```python
from build123d import *

# Parameters (mm, degrees)
ESTRUSIONE_ESTRUSIONE1_DEPTH = 5
SCHIZZO2_R                   = 2
TAGLIO_ESTRUSIONE1_DEPTH     = 5
SCHIZZO4_R                   = 4.75
TAGLIO_ESTRUSIONE2_DEPTH     = 10


with BuildPart() as part:
    # Schizzo1 → Estrusione-Estrusione1 (new body)
    with BuildSketch(Plane.XY):
        with BuildLine():
            Line((0, 145), (0, 120))
            ThreePointArc((0, 120), (-20.689655172, 118.2029533), (-40.759639069, 112.865636147))
            Line((-40.759639069, 112.865636147), (-49.251230542, 136.379310345))
            ThreePointArc((-49.251230542, 136.379310345), (-25, 142.828568571), (0, 145))
        make_face()
    extrude(amount=ESTRUSIONE_ESTRUSIONE1_DEPTH)

    # Schizzo2 → Taglio-Estrusione1 (cut)
    with BuildSketch(Plane.XY.offset(5)):
        with Locations((-38.032134419, 134.73513555)):
            Circle(SCHIZZO2_R)
        with Locations((-9.993620414, 139.642857143)):
            Circle(SCHIZZO2_R)
    extrude(amount=-TAGLIO_ESTRUSIONE1_DEPTH, mode=Mode.SUBTRACT)

    # Raccordo1
    # an asymmetric fillet: 20, 15 mm, written as the material it takes off along each edge
    with BuildSketch(Plane(origin=(-40.759639069, 112.865636147, -44.567563269), x_dir=(-0.3396636589081028, 0.9405469678953624, 0), z_dir=(0, 0, 1))) as raccordo1_piece_1:
        with BuildLine():
            Bezier((13.510299228, 0), (1.338953576, 0), (-1.324178464, -17.777777778), weights=[1, 0.757676761, 1])
            ThreePointArc((-1.324178464, -17.777777778), (-0.331502507, -8.913512654), (0, 0))
            Line((0, 0), (13.510299228, 0))
        make_face()
    extrude(amount=94.135126538, mode=Mode.SUBTRACT)

    # Raccordo2
    # an asymmetric fillet: 20, 15 mm, written as the material it takes off along each edge
    with BuildSketch(Plane(origin=(0, 120, -44.567563269), x_dir=(-0.9972374791061684, -0.07427927211527091, 0), z_dir=(0, 0, 1))) as raccordo2_piece_1:
        with BuildLine():
            Bezier((17.827025308, 0), (-0.099456497, -1.335254689), (-1.003535193, -13.472976744), weights=[1, 0.757676761, 1])
            Line((-1.003535193, -13.472976744), (0, 0))
            ThreePointArc((0, 0), (8.913512654, -0.331502507), (17.827025308, 0))
        make_face()
    extrude(amount=94.135126538, mode=Mode.SUBTRACT)

    # Schizzo4 → Taglio-Estrusione2 (cut)
    with BuildSketch(Plane.XY.offset(5)):
        with Locations((-22.24137931, 127.068174798)):
            Circle(SCHIZZO4_R)
    extrude(amount=-TAGLIO_ESTRUSIONE2_DEPTH, mode=Mode.SUBTRACT)


solid = part.part
```
Source: CAD feature listing. Evaluate the final solid. Frame: model axes, mm. Round coordinates to 2 decimals unless told otherwise and drop trailing zeros. Loops run counter-clockwise (first coordinate to the right, second up) from the corner with the lowest first, then second, coordinate; pieces in that order, holes last.
1. Mould query, pull axis Y, two halves, no side actions, for faces 1 (the cylindrical face through (-9.07, 137.87, 2.54)), 2 (the cylindrical face through (-38.29, 136.72, 2.54)), 3 (the flat face through (-24, 134, 0)), 4 (the cylindrical face through (-20.65, 118.21, 2.46)). Classes: released by +Y, released by -Y, zero draft, split by the parting line, or undercut.
2. Ray query, L1, parallel to X at y = 131, z = 0.65; L2, parallel to Y at x = -18, z = 4.7; L3, parallel to X at y = 130.5, z = 2.15. Return the intervals inside material, ascending.
3. Section query A-A on x = -19. Output: boundary loops of the cut face in (y, z), and give its area (3 significant figures).
4. Section query C-C on z = 3.85. Give the number of separate pieces and of enclosed holes in the cut face, and give its area (3 significant figures).
5. Section query B-B on y = 139. Output: boundary loops of the cut face in (x, z).
Answers below:
1. face 1: undercut
1. face 2: undercut
1. face 3: zero draft
1. face 4: released by -Y
2. L1: x = -47.31 to -24.91, -19.58 to -0.33
2. L2: y = 118.64 to 124.93, 129.21 to 143.88
2. L3: x = -47.13 to -25.53, -18.96 to -0.47
3. outline: (118.49, 0) - (123.6, 0) - (123.6, 5) - (118.49, 5) - close; (130.54, 0) - (143.75, 0) - (143.75, 5) - (130.54, 5) - close
3. area: 91.6 mm2
4. separate pieces: 1
4. enclosed holes: 3
4. area: 947 mm2
5. outline: (-41.28, 0) - (-11.89, 0) - (-11.89, 5) - (-41.28, 5) - close; (-8.1, 0) - (0, 0) - (0, 5) - (-8.1, 5) - close
